```python
from build123d import *

# Parameters (mm, degrees)
SKETCH1_W           = 47
SKETCH1_H           = 131
BOSS_EXTRUDE1_DEPTH = 4.9
BOSS_EXTRUDE2_DEPTH = 50
SKETCH2_R           = 1.95
CUT_EXTRUDE1_DEPTH  = 6


with BuildPart() as part:
    # Sketch1 → Boss-Extrude1 (new body)
    with BuildSketch(Plane(origin=(0, 0, 0), x_dir=(1, 0, 0), z_dir=(0, 1, 0))):
        Rectangle(SKETCH1_W, SKETCH1_H)
    extrude(amount=BOSS_EXTRUDE1_DEPTH)

    # Sketch3 → Boss-Extrude2 (add)
    with BuildSketch(Plane.XY.offset(65.5)):
        Polygon((-4.9, 0), (4.9, 0), (4.9, -5.2), (8.8, -5.2), (4.9, -10), (-4.9, -10), (-8.8, -5.2), (-4.9, -5.2), align=None)
    extrude(amount=-BOSS_EXTRUDE2_DEPTH)

    # Sketch2 → Cut-Extrude1 (cut)
    with BuildSketch(Plane(origin=(0, 4.9, 0), x_dir=(1, 0, 0), z_dir=(0, 1, 0))):
        with Locations((0, 62)):
            Circle(SKETCH2_R)
        with Locations((0, -62)):
            Circle(SKETCH2_R)
    extrude(amount=-CUT_EXTRUDE1_DEPTH, mode=Mode.SUBTRACT)


solid = part.part
```
Read the model definition and answer for the solid it produces. Units are mm, in the model's axes. A direction names the side the tool comes from. Round coordinates to 2 decimals unless told otherwise and drop trailing zeros. Write each loop counter-clockwise with the first axis right and the second up, starting at its lowest first coordinate (ties: lowest second). Pieces come first, ordered by that corner, then holes. Notation, with made-up numbers: M 10.5,-6 L 30.5,-6 A19 cw 30.5,4 Z; hole C 78.5,7.5 d11. An arc over 180 degrees is marked long. One line per item, written item: value.
Q1. Find section B-B on x = 0. Write down the section's boundary in (y, z).
Data:
outline: M -10,15.5 L 0,15.5 L 0,-60.05 L 4.9,-60.05 L 4.9,60.05 L -1.1,60.05 L -1.1,63.95 L 4.9,63.95 L 4.9,65.5 L -10,65.5 Z; M 0,-65.5 L 4.9,-65.5 L 4.9,-63.95 L 0,-63.95 Z
Q2. Find section C-C on z = 62. Write down the section's boundary in (x, y), plus the area to 3 significant figures.
Data:
outline: M -23.5,0 L -4.9,0 L -4.9,-5.2 L -8.8,-5.2 L -4.9,-10 L 4.9,-10 L 8.8,-5.2 L 4.9,-5.2 L 4.9,0 L 23.5,0 L 23.5,4.9 L 1.95,4.9 L 1.95,-1.1 L -1.95,-1.1 L -1.95,4.9 L -23.5,4.9 Z
area: 324 mm2
Q3. For a pull along Z with two mould halves and no side action, classify faces 1 (the flat face through (-6.823, -7.634, 40.85)), 2 (the cylindrical face through (-0.254, 2.484, -63.933)), 3 (the flat face through (0, 2, -65.5)) as +Z half, -Z half, draft (parallel to the pull), parting line (faces both ways), or undercut.
Data:
face 1: draft
face 2: undercut
face 3: -Z half
Q4. Flat-ended cylindrical pins translate along their axes: pin 1 Ø1 at (x, y) = (7, -1) entering from +Z; pin 2 Ø3 at (x, z) = (0, 62) entering from +Y; pin 3 Ø23.5 at (x, z) = (-9.5, 27.5) entering from -Y; pin 4 Ø6 at (x, y) = (5.5, -7.5) entering from -Z. Find the tip coordinate at first contact, or state that the pin passes through.
Data:
pin 1: through
pin 2: y = -1.1
pin 3: y = -10
pin 4: z = 15.5
Q5. Straight lines are drawn through the part: line 1 (Z direction, x = 0, y = 1.9); line 2 (X direction, y = 1.5, z = -62); line 3 (Y direction, x = 14, z = -52.5). For each, find the intervals that lie inside material, in ascending order. Write a range as [from, to].
Data:
line 1: [-65.5, -63.95], [-60.05, 60.05], [63.95, 65.5]
line 2: [-23.5, -1.95], [1.95, 23.5]
line 3: [0, 4.9]
Q6. Which of the six approach directions +Z, -Z, +X, -X, +Y, -Y give full straight-line access (tool end or side, diameter ignored) to faces 4 (the flat face through (-4.9, -3, 41)), 5 (the flat face through (0, -5, 15.5)), 6 (the flat face through (4.9, -3, 41)), 7 (the flat face through (0, -1.1, 62))?
Data:
face 4: +Z, -Z, -X
face 5: -Z, +X, -X, -Y
face 6: +Z, -Z, +X
face 7: +Y
Q7. Find section A-A on z = -62. Write down the section's boundary in (x, y), plus the area to 3 significant figures.
Data:
outline: M -23.5,0 L -1.95,0 L -1.95,4.9 L -23.5,4.9 Z; M 1.95,0 L 23.5,0 L 23.5,4.9 L 1.95,4.9 Z
area: 211 mm2
Q8. Find section D-D on x = -11. Write down the section's boundary in (y, z).
Data:
outline: M 0,-65.5 L 4.9,-65.5 L 4.9,65.5 L 0,65.5 Z
